The figure shows three views and two pictorial views of one solid part (mm, origin at its lowest corner). Answer the questions. Give positions to 0.01 mm unless a question says otherwise; leave off trailing zeros. Order: outer loops, then holes, each group sorted by start corner. A loop starts at its lowest first (then second) coordinate and runs counter-clockwise, first axis right, second up. Notation, with made-up numbers: (33, 22) - (72, 22) arc R17 ccw to (72, 47) - close; hole circle Ø1 at (66.5, -34.75). An arc over 180 degrees is marked (long way). Answer as CSV lines item,"result". Start each with the question number.
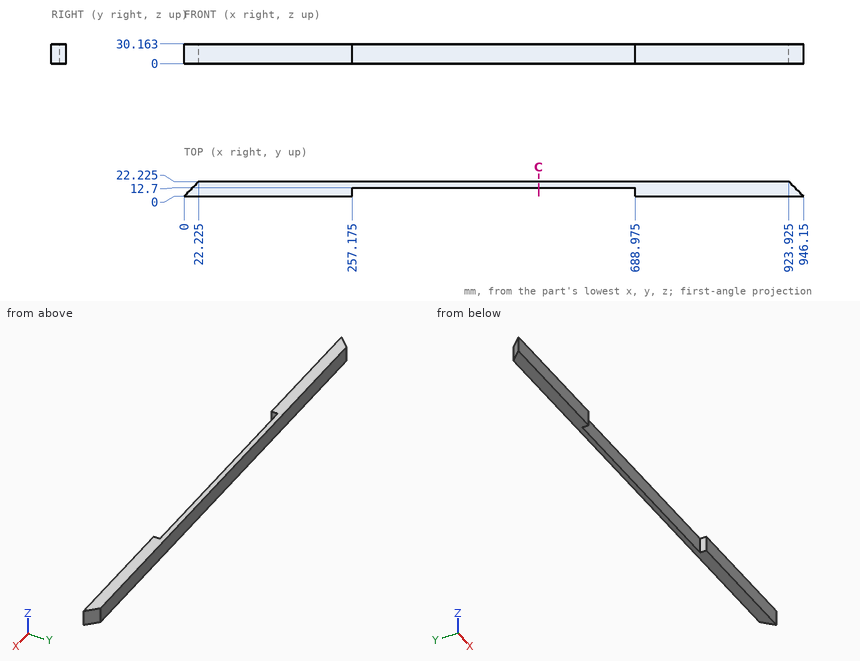
(1) Section C-C, the plane x = 541.5 is taken. Write down the section's boundary in (y, z) (1 decimal), and give its area (3 significant figures).
(2) Flat-ended cylindrical pins translate along their axes: pin 1 Ø6.5 at (y, z) = (7, 19) entering from +X; pin 2 Ø1.5 at (y, z) = (7, 6.5) entering from +X; pin 3 Ø1 at (x, z) = (565, 14) entering from -Y; pin 4 Ø12 at (x, z) = (724, 15.5) entering from -Y. Find the tip coordinate at first contact, or state that the pin passes through.
(3) Straight lines are drawn through the part: line 1 (Y direction, x = 385, z = 3) (1 decimal); line 2 (X direction, y = 18, z = 24.5); line 3 (X direction, y = 13.5, z = 12.5). For each, find the intervals that lie inside material, in ascending order. Write a range as [from, to].
Checks:
1,outline,"(12.7, 0) - (22.2, 0) - (22.2, 30.2) - (12.7, 30.2) - close"
1,area,"287 mm²"
2,pin 1,"stops at x = 942.4"
2,pin 2,"stops at x = 939.9"
2,pin 3,"stops at y = 12.7"
2,pin 4,"stops at y = 0"
3,line 1,"y = [12.7, 22.2]"
3,line 2,"x = [18, 928.15]"
3,line 3,"x = [13.5, 932.65]"
